from build123d import *

# Parameters (mm, degrees)
F0_W     = 40
F0_H     = 40
F1_DEPTH = 40


with BuildPart() as f1:
    # F0 (on Front) → F1 (new body)
    with BuildSketch(Plane.XZ):
        with Locations((-40, 80)):
            Rectangle(F0_W, F0_H)
        with Locations((-40, 40)):
            Rectangle(F0_W, F0_H)
        with Locations((-40, 0)):
            Rectangle(F0_W, F0_H)
        with Locations((-40, -40)):
            Rectangle(F0_W, F0_H)
        with Locations((-40, -80)):
            Rectangle(F0_W, F0_H)
        Polygon((20, -20), (20, 20), (0, 20), (-20, 20), (-20, -20), (0, -20), align=None)
        Polygon((35, 0), (40, 20), (20, 20), (20, -20), (40, -20), align=None)
        Polygon((40, -20), (20, -20), (20, -60), (50, -60), align=None)
        Polygon((50, -60), (20, -60), (20, -100), (60, -100), align=None)
        Polygon((20, -60), (20, -20), (0, -20), (10, -60), align=None)
        Polygon((20, -100), (20, -60), (10, -60), align=None)
        Polygon((20, 20), (20, 60), (10, 60), (0, 20), align=None)
        Polygon((40, 20), (50, 60), (20, 60), (20, 20), align=None)
        Polygon((50, 60), (60, 100), (20, 100), (20, 60), align=None)
        Polygon((20, 60), (20, 100), (10, 60), align=None)
    extrude(amount=F1_DEPTH)


solid = f1.part
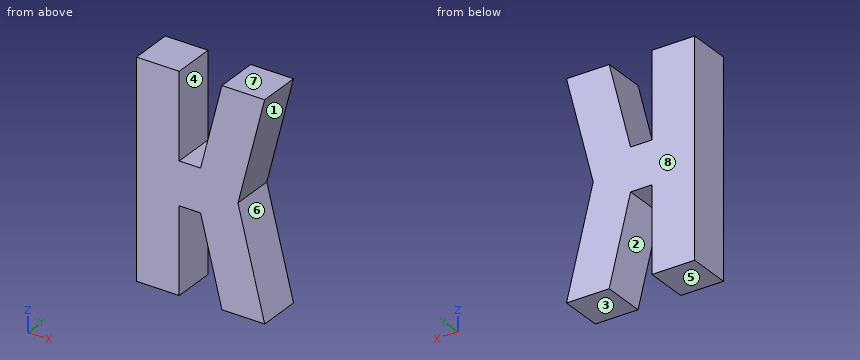
Model file for the job. Use its own axes, mm. Face numbers are marked on the shaded views. A direction names the side the tool comes from. Give positions to 0.01 mm unless a question says otherwise; leave off trailing zeros. Loops run counter-clockwise (first coordinate to the right, second up) from the corner with the lowest first, then second, coordinate; pieces in that order, holes last.
1) Wall check: line 1 (X direction, y = -15.5, z = 51.5) (3 decimals); line 2 (X direction, y = -1.5, z = 25); line 3 (Z direction, x = -19, y = -14). Give the ranges that are in metal, low to high.
2) Tool access for the marked faces 1, 2, 3 and 4: list every direction of +Z, -Z, +X, -X, +Y, -Y with a clear straight run to the whole face (end or side of a thin tool).
3) Saw through at D-D (z = 14). Write the cut outline in (x, y), plus the area to 3 significant figures.
4) Saw through at A-A (x = 48). Write the cut outline in (y, z).
5) Pull direction Z, two halves, no side cores. Call the marked faces 5, 6, 7 and 8: +Z half, -Z half, draft (parallel to the pull), parting line (faces both ways), or undercut.
6) Saw through at C-C (y = -36.5). Write the cut outline in (x, z).
7) Saw through at B-B (z = -46). Write the cut outline in (x, y), plus the area to 3 significant figures.
8) Flat gauge pins, fed straight in: pin 1 Ø6 at (x, y) = (-8, -26) entering from -Z; pin 2 Ø2 at (x, y) = (-7, -30) entering from +Z; pin 3 Ø20 at (y, z) = (-15, -55) entering from +X. Where does each tip first touch, or does it go through?
Answer block:
1. line 1: x = -60 to -20, 7.875 to 47.875
1. line 2: x = -60 to -20, 1.25 to 41.25
1. line 3: z = -20 to 20
2. face 1: +X, +Y, -Y
2. face 2: -Z, +Y, -Y
2. face 3: -Z, +X, -X, +Y, -Y
2. face 4: +Z, +Y, -Y
3. outline: (-60, -40) - (38.5, -40) - (38.5, 0) - (-60, 0) - close
3. area: 3,940 mm2
4. outline: (-40, -100) - (0, -100) - (0, -52) - (-40, -52) - close; (-40, 52) - (0, 52) - (0, 100) - (-40, 100) - close
5. face 5: -Z half
5. face 6: undercut
5. face 7: +Z half
5. face 8: draft
6. outline: (-60, -100) - (-20, -100) - (-20, -20) - (0, -20) - (20, -100) - (60, -100) - (35, 0) - (60, 100) - (20, 100) - (0, 20) - (-20, 20) - (-20, 100) - (-60, 100) - close
7. outline: (-60, -40) - (-20, -40) - (-20, 0) - (-60, 0) - close; (6.5, -40) - (46.5, -40) - (46.5, 0) - (6.5, 0) - close
7. area: 3,200 mm2
8. pin 1: stops at z = -20
8. pin 2: stops at z = 20
8. pin 3: stops at x = 51.25
